Autodesk Inventor part; units mm, degrees
ref_plane "YZ Plane" through (0, 0, 0) normal (1, 0, 0) x (0, 1, 0)
ref_plane "XZ Plane" through (0, 0, 0) normal (0, 1, 0) x (-1, 0, 0)
ref_plane "XY Plane" through (0, 0, 0) normal (0, 0, 1) x (1, 0, 0)
sketch "Sketch1" plane through (0, 0, 0) normal (0, 0, 1) x (1, 0, 0)
  circle A0 centre (0, 0) radius 4
  line L0 (2.1406, -3.379) -> (2.1439, -3.379)
  point P0 (-2.1406, -3.379)
  dimension "d0" = 8
extrude "Extrusion1" add sketch "Sketch1" along normal blind 75
sketch "Sketch2" plane through (0, 0, 0) normal (0, 0, -1) x (-1, 0, 0)
  circle A0 centre (0, 0) radius 4
  line L0 (0, -7.5056) -> (-6.5, -3.7528)
  line L1 (-6.5, -3.7528) -> (-6.5, 3.7528)
  line L2 (-6.5, 3.7528) -> (0, 7.5056)
  line L3 (0, 7.5056) -> (6.5, 3.7528)
  line L4 (6.5, 3.7528) -> (6.5, -3.7528)
  line L5 (6.5, -3.7528) -> (0, -7.5056)
  dimension "d4" = 13
extrude "Extrusion2" add sketch "Sketch2" against normal blind 4
properties part number "8mm-rod" material "Iron, Cast"
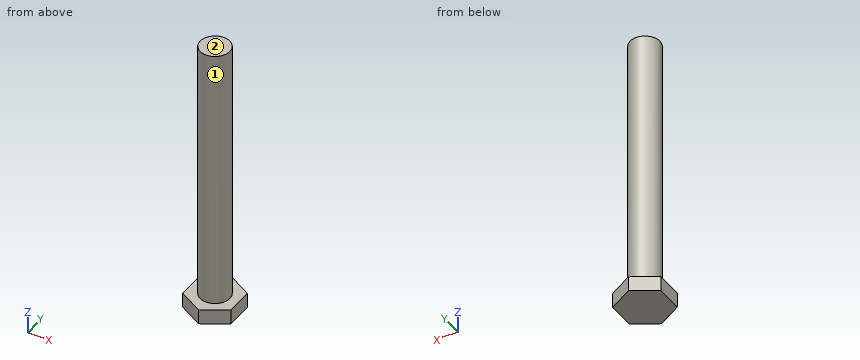
Could you check a few things on this model? Use its own coordinates, in mm. Face numbers are marked on the shaded views. A direction names the side the tool comes from. Give positions to 0.01 mm unless a question says otherwise; leave off trailing zeros. Order: outer loops, then holes, each group sorted by start corner. A loop starts at its lowest first (then second) coordinate and runs counter-clockwise, first axis right, second up.
Item 1: I need wall thicknesses on line 1 (Z direction, x = 3, y = -5); line 2 (Y direction, x = -0.25, z = 26); line 3 (X direction, y = -1.5, z = 40.5). Which ranges of each line are inside material? Lowest first, please.
Item 2: If we section it at B-B, the plane x = 2.25: Write out the boundary of the cut face in (y, z).
Item 3: I'm going to push flat-ended pins straight in: pin 1 (6 mm diameter, centred on y = 2.5, z = 11, fed in from -X); pin 2 (2 mm diameter, centred on x = 4.5, z = 42, fed in from +Y); pin 3 (3 mm diameter, centred on y = 3, z = 9.5, fed in from -X). Where does each tip first touch, or does it pass through?
Item 4: For the marked faces 1 and 2, which set-ups out of +Z, -Z, +X, -X, +Y, -Y let a thin tool reach every point of the face, with its end or its side?
Item 5: If we section it at A-A, the plane y = 0: Write out the boundary of the cut face in (x, z), plus the area to 3 significant figures.
Item 6: If we section it at C-C, the plane z = 12: Write out the boundary of the cut face in (x, y).
Item 7: If we section it at D-D, the plane y = 6.75: Write out the boundary of the cut face in (x, z).
Values:
1. line 1: z = 0 to 4
1. line 2: y = -3.99 to 3.99
1. line 3: x = -3.71 to 3.71
2. outline: (-6.21, 0) - (6.21, 0) - (6.21, 4) - (3.31, 4) - (3.31, 75) - (-3.31, 75) - (-3.31, 4) - (-6.21, 4) - close
3. pin 1: stops at x = -4
3. pin 2: stops at y = 1.94
3. pin 3: stops at x = -3.71
4. face 1: +Z
4. face 2: +Z, +X, -X, +Y, -Y
5. outline: (-6.5, 0) - (6.5, 0) - (6.5, 4) - (4, 4) - (4, 75) - (-4, 75) - (-4, 4) - (-6.5, 4) - close
5. area: 620 mm2
6. outline: circle Ø8 at (0, 0)
7. outline: (-1.31, 0) - (1.31, 0) - (1.31, 4) - (-1.31, 4) - close
